Could you check a few things on this model? Use its own coordinates, in mm. Face numbers are marked on the shaded views. Coordinates: 2 decimals unless noted, no trailing zeros. Order: outer loops, then holes, each group sorted by start corner. A loop starts at its lowest first (then second) coordinate and runs counter-clockwise, first axis right, second up. Notation, with made-up numbers: (70, 29) - (107, 29) arc R31 cw to (107, 60) - close; hole circle Ø8 at (60.25, 60). An arc over 180 degrees is marked (long way). Answer as CSV lines item,"result". Start each with the question number.
1. I want a section at C-C, the plane y = -3.25. List the corners of the cut face in (x, z) for me, and give its area (3 significant figures).
2. I want a section at B-B, the plane x = -5. List the corners of the cut face in (y, z) for me.
3. I want a section at D-D, the plane x = -1. List the corners of the cut face in (y, z) for me, and give its area (3 significant figures).
4. For pin 1 (3 mm diameter, centred on x = -1.5, y = -7, fed in from -Z); pin 2 (0.7 mm diameter, centred on x = 1, z = -9.5, fed in from +Y); pin 3 (3.5 mm diameter, centred on y = 3, z = -5.5, fed in from -X), each with a flat end and sliding along its axis, tell me the tip position at first contact or that it passes through.
5. Thinking about a two-plate mould opening in X: for the marked faces 1, 2, 3 and 4, which applies, released by +X, released by -X, zero draft, split by the parting line, or undercut?
6. I want a section at A-A, the plane z = -0.5. List the corners of the cut face in (x, y) for me.
7. I need wall thicknesses on probe 1 along X at (y, z) = (-7, 5); probe 2 along Y at (x, z) = (1.5, -8); probe 3 along X at (y, z) = (1.25, -3.5). Which ranges of each line are inside material? Lowest first, please.
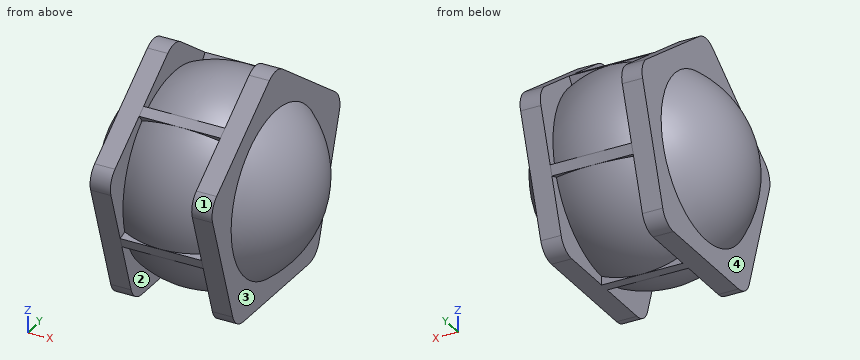
from build123d import *

# Parameters (mm, degrees)
F4_DEPTH  = 1
F7_DEPTH  = 1
F8_R      = 2
F10_DEPTH = 8


with BuildPart() as f1:
    # F0 (on Right) → F1 (revolve)
    with BuildSketch(Plane.YZ):
        with BuildLine():
            Line((0, -10), (0, 10))
            ThreePointArc((0, 10), (-10, 0), (0, -10))
        make_face()
    revolve(axis=Axis((0, 0, 0), (0, 0, -1)))

    # F3 (on offset) → F4 (join, symmetric)
    with BuildSketch(Plane.YZ.offset(5)):
        Polygon((-7.2654252801, -10), (7.2654252801, -10), (11.7557050458, 3.8196601125), (0, 12.360679775), (-11.7557050458, 3.8196601125), align=None)
    extrude(amount=F4_DEPTH, both=True)

    # F6 (on offset) → F7 (join, symmetric)
    with BuildSketch(Plane.YZ.offset(-5)):
        Polygon((-7.2654252801, -10), (7.2654252801, -10), (11.7557050458, 3.8196601125), (0, 12.360679775), (-11.7557050458, 3.8196601125), align=None)
    extrude(amount=F7_DEPTH, both=True)

    # F8
    f8_edges = [f1.edges().sort_by_distance(p)[0] for p in [
        (-5, -11.755705, 3.81966),
        (-5, 0, 12.36068),
        (5, 0, 12.36068),
        (5, -11.755705, 3.81966),
        (-5, -7.265425, -10),
        (5, -7.265425, -10),
        (5, 11.755705, 3.81966),
        (-5, 11.755705, 3.81966),
        (5, 7.265425, -10),
        (-5, 7.265425, -10),
    ]]
    fillet(f8_edges, radius=F8_R)

    # F9 (on face) → F10 (join)
    with BuildSketch(Plane.YZ.offset(-4)):
        with BuildLine():
            ThreePointArc((-5.783626767, 7.1098285085), (-5.387140822, 7.4147632305), (-4.9746097726, 7.6976137608))
            Line((-4.9746097726, 7.6976137608), (-5.4733440257, 8.3840625699))
            Line((-5.4733440257, 8.3840625699), (-6.2823610201, 7.7962773176))
            Line((-6.2823610201, 7.7962773176), (-5.783626767, 7.1098285085))
        make_face()
        with BuildLine():
            Line((5.4733440257, 8.3840625699), (4.9746097726, 7.6976137608))
            ThreePointArc((4.9746097726, 7.6976137608), (5.387140822, 7.4147632305), (5.783626767, 7.1098285085))
            Line((5.783626767, 7.1098285085), (6.2823610201, 7.7962773176))
            Line((6.2823610201, 7.7962773176), (5.4733440257, 8.3840625699))
        make_face()
        with BuildLine():
            Line((9.6650736601, -2.6146416856), (8.8581046872, -2.3524415721))
            ThreePointArc((8.8581046872, -2.3524415721), (8.7165769522, -2.8321875355), (8.5490876929, -3.3034980884))
            Line((8.5490876929, -3.3034980884), (9.3560566658, -3.5656982019))
            Line((9.3560566658, -3.5656982019), (9.6650736601, -2.6146416856))
        make_face()
        with BuildLine():
            ThreePointArc((0.5, -9.1515026089), (0, -9.1651513899), (-0.5, -9.1515026089))
            Line((-0.5, -9.1515026089), (-0.5, -10))
            Line((-0.5, -10), (0.5, -10))
            Line((0.5, -10), (0.5, -9.1515026089))
        make_face()
        with BuildLine():
            ThreePointArc((-8.5490876929, -3.3034980884), (-8.7165769522, -2.8321875355), (-8.8581046872, -2.3524415721))
            Line((-8.8581046872, -2.3524415721), (-9.6650736601, -2.6146416856))
            Line((-9.6650736601, -2.6146416856), (-9.3560566658, -3.5656982019))
            Line((-9.3560566658, -3.5656982019), (-8.5490876929, -3.3034980884))
        make_face()
    extrude(amount=F10_DEPTH)


solid = f1.part
Solved:
1,outline,"(-6, -10) - (-4, -10) - (-4, -8.57) arc R9.46 ccw to (4, -8.57) - (4, -10) - (6, -10) - (6, -7.31) arc R9.46 ccw to (6, 7.31) - (6, 10) - (4, 10) - (4, 8.57) arc R9.46 ccw to (-4, 8.57) - (-4, 10) - (-6, 10) - (-6, 7.31) arc R9.46 ccw to (-6, -7.31) - close"
1,area,"297 mm2"
2,outline,"(-11.31, 2.44) - (-7.71, -8.62) arc R2 ccw to (-5.81, -10) - (5.81, -10) arc R2 ccw to (7.71, -8.62) - (11.31, 2.44) arc R2 ccw to (10.58, 4.67) - (1.18, 11.51) arc R2 ccw to (-1.18, 11.51) - (-10.58, 4.67) arc R2 ccw to start"
3,outline,"(-9.67, -2.61) - (-9.36, -3.57) - (-9.3, -3.55) arc R9.95 ccw to (-0.5, -9.94) - (-0.5, -10) - (0.5, -10) - (0.5, -9.94) arc R9.95 ccw to (9.3, -3.55) - (9.36, -3.57) - (9.67, -2.61) - (9.61, -2.6) arc R9.95 ccw to (6.25, 7.75) - (6.28, 7.8) - (5.47, 8.38) - (5.44, 8.33) arc R9.95 ccw to (-5.44, 8.33) - (-5.47, 8.38) - (-6.28, 7.8) - (-6.25, 7.75) arc R9.95 ccw to (-9.61, -2.6) - close"
3,area,"311 mm2"
4,pin 1,"stops at z = -8.24"
4,pin 2,"stops at y = 3.91"
4,pin 3,"stops at x = -8.92"
5,face 1,"zero draft"
5,face 2,"undercut"
5,face 3,"released by +X"
5,face 4,"released by -X"
6,outline,"(-6, -10.35) - (-4, -10.35) - (-4, -9.15) arc R9.99 ccw to (4, -9.15) - (4, -10.35) - (6, -10.35) - (6, -7.98) arc R9.99 ccw to (6, 7.98) - (6, 10.35) - (4, 10.35) - (4, 9.15) arc R9.99 ccw to (-4, 9.15) - (-4, 10.35) - (-6, 10.35) - (-6, 7.98) arc R9.99 ccw to (-6, -7.98) - close"
7,probe 1,"x = -6 to 6"
7,probe 2,"y = -5.81 to 5.81"
7,probe 3,"x = -9.28 to 9.28"
